Verification items for this drawing (mm, ordinates from the low corner). Coordinates: 2 decimals unless noted, no trailing zeros. Order: outer loops, then holes, each group sorted by start corner. A loop starts at its lowest first (then second) coordinate and runs counter-clockwise, first axis right, second up.
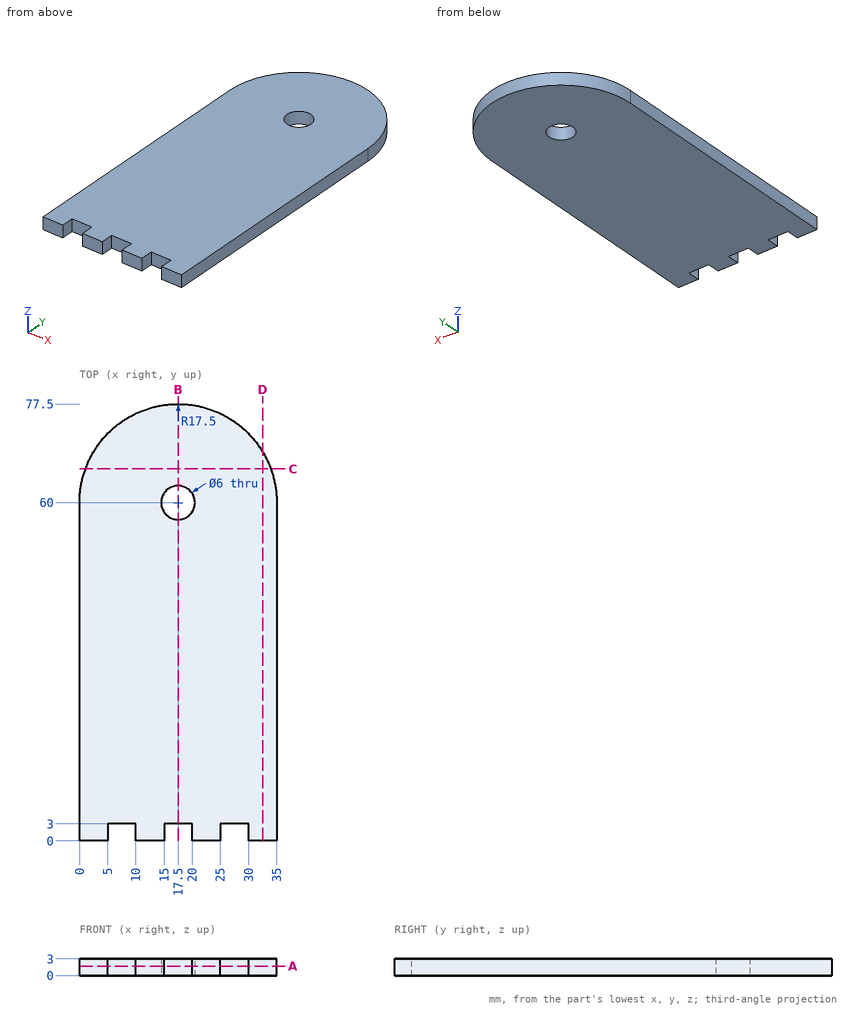
(1) Thickness scan on probe 1 along Y at (x, z) = (17.5, 0.9); probe 2 along Y at (x, z) = (29.5, 0.3); probe 3 along Y at (x, z) = (4.5, 1.1). Record the ranges inside material, lowest first.
Filled in:
probe 1: y = 3 to 57, 63 to 77.5
probe 2: y = 3 to 72.74
probe 3: y = 0 to 71.72
(2) Go/stop test with flat-tipped pins: P1, Ø3, axis at x = 30.5, y = 16, coming from the -Z side; P2, Ø1.5, axis at x = 16.5, z = 2, coming from the -Y side. Record where each tip stops, or that it passes through.
Filled in:
P1: stops at z = 0
P2: stops at y = 3
(3) Cross-section at C-C (y = 66). Enter the section's corners in (x, z), and give its area (3 significant figures).
Filled in:
outline: (1.06, 0) - (33.94, 0) - (33.94, 3) - (1.06, 3) - close
area: 98.6 mm2
(4) Cross-section at A-A (z = 1.7). Enter the section's corners in (x, y).
Filled in:
outline: (0, 0) - (5, 0) - (5, 3) - (10, 3) - (10, 0) - (15, 0) - (15, 3) - (20, 3) - (20, 0) - (25, 0) - (25, 3) - (30, 3) - (30, 0) - (35, 0) - (35, 60) arc R17.5 ccw to (0, 60) - close; hole circle Ø6 at (17.5, 60)
(5) Cross-section at D-D (x = 32.5). Enter the section's corners in (y, z), and give its area (3 significant figures).
Filled in:
outline: (0, 0) - (69.01, 0) - (69.01, 3) - (0, 3) - close
area: 207 mm2
(6) Cross-section at B-B (x = 17.5). Enter the section's corners in (y, z), and give its area (4 significant figures).
Filled in:
outline: (3, 0) - (57, 0) - (57, 3) - (3, 3) - close; (63, 0) - (77.5, 0) - (77.5, 3) - (63, 3) - close
area: 205.5 mm2
